from build123d import *

# Parameters (mm, degrees)
F0_W      = 63.5
F0_H      = 64
F1_DEPTH  = 2.5
F3_DEPTH  = 12
F5_DEPTH  = 10
F6_R      = 2.2
F7_R      = 2
F8_R      = 1.95
F9_DEPTH  = 1.5
F10_R     = 1.49999
F11_R     = 1.95
F12_DEPTH = 1.5
F13_R     = 1.49999


# Not quite as in the source:
# - a fillet or chamfer is up to 0.001 mm smaller than in the source, because OpenCascade refuses the exact size


with BuildPart() as f1:
    # F0 (on Top) → F1 (new body)
    with BuildSketch(Plane.XY):
        Rectangle(F0_W, F0_H)
    extrude(amount=F1_DEPTH)

    # F2 (on face) → F3 (join)
    with BuildSketch(Plane.XY.offset(2.5)):
        Polygon((-25.75, 32), (-31.75, 32), (-31.75, -32), (31.75, -32), (31.75, 32), (25.75, 32), (25.75, -26), (-25.75, -26), align=None)
    extrude(amount=F3_DEPTH)

    # F4 (on face) → F5 (join)
    with BuildSketch(Plane.XY.offset(14.5)):
        Polygon((-28.9, 32), (-31.75, 32), (-31.75, -32), (31.75, -32), (31.75, 32), (28.9, 32), (28.9, -29.15), (-28.9, -29.15), align=None)
    extrude(amount=F5_DEPTH)

    # F6
    f6_edges = [f1.edges().sort_by_distance(p)[0] for p in [
        (-28.9, -29.15, 19.5),
        (28.9, -29.15, 19.5),
    ]]
    fillet(f6_edges, radius=F6_R)

    # F7
    f7_edges = [f1.edges().sort_by_distance(p)[0] for p in [
        (-31.75, 0, 24.5),
        (0, -32, 24.5),
        (31.75, 0, 24.5),
    ]]
    fillet(f7_edges, radius=F7_R)

    # F8 (on face) → F9 (join)
    with BuildSketch(Plane.YZ.offset(-28.9)):
        with Locations((0, 19.5)):
            Circle(F8_R)
    extrude(amount=F9_DEPTH)

    # F10 (radius 1.5 in the source; OpenCascade refuses exactly that, so slightly less here)
    f10_edges = [f1.edges().sort_by_distance(p)[0] for p in [
        (-27.4, -1.95, 19.5),
    ]]
    fillet(f10_edges, radius=F10_R)

    # F11 (on face) → F12 (join)
    with BuildSketch(Plane(origin=(28.9, 0, 0), x_dir=(0, -1, 0), z_dir=(-1, 0, 0))):
        with Locations((0, 19.5)):
            Circle(F11_R)
    extrude(amount=F12_DEPTH)

    # F13 (radius 1.5 in the source; OpenCascade refuses exactly that, so slightly less here)
    f13_edges = [f1.edges().sort_by_distance(p)[0] for p in [
        (27.4, 1.95, 19.5),
    ]]
    fillet(f13_edges, radius=F13_R)


solid = f1.part
Work out the finished part from the listing and answer in its coordinate system (mm). A direction names the side the tool comes from. Coordinates: 2 decimals unless noted, no trailing zeros. Write each loop counter-clockwise with the first axis right and the second up, starting at its lowest first coordinate (ties: lowest second). Pieces come first, ordered by that corner, then holes. Notation, with made-up numbers: M 27.25,41.25 L 37.25,41.25 A14 cw 37.25,48.25 Z; hole C -28,2.5 d8. An arc over 180 degrees is marked long. Use one line per item in the form item = value. Start each with the question number.
1. The part is cut by section B-B (z = 12.5). Give the vertices of the cut face in (x, y).
2. The part is cut by section C-C (y = -9). Give the vertices of the cut face in (x, z), plus the area to 3 significant figures.
3. Straight lines are drawn through the part: probe 1 along X at (y, z) = (25, 17.75); probe 2 along X at (y, z) = (2.5, 4); probe 3 along Y at (x, z) = (-2.5, 14.25). For each, find the intervals that lie inside material, in ascending order. Write a range as from..to.
4. A tool of negligible diameter and unlimited length cuts with its end or side. For faces 1 (the face through (31.75, 0, 11)), 2 (the face through (0, 3, 2.5)), 3 (the face through (-28.24, -28.52, 19.57)), from which of +Z, -Z, +X, -X, +Y, -Y can it reach the whole face along a straight path? Write none if from no direction.
5. Each of these flat-tipped pins is pushed along its axis until it touches: P1, Ø12, axis at x = 15, z = 4, coming from the +Y side; P2, Ø6, axis at x = 4.5, z = 10, coming from the +Y side; P3, Ø10, axis at x = 19.5, y = -0.5, coming from the +Z side; P4, Ø3, axis at x = -9, z = 20, coming from the +Y side. Where does it stop, or does it pass through?
6. The part is cut by section A-A (x = 22). Give the vertices of the cut face in (y, z).
Evaluation:
q1.outline = M -31.75,-32 L 31.75,-32 L 31.75,32 L 25.75,32 L 25.75,-26 L -25.75,-26 L -25.75,32 L -31.75,32 Z
q2.outline = M -31.75,0 L 31.75,0 L 31.75,22.5 A2 ccw 29.75,24.5 L 28.9,24.5 L 28.9,14.5 L 25.75,14.5 L 25.75,2.5 L -25.75,2.5 L -25.75,14.5 L -28.9,14.5 L -28.9,24.5 L -29.75,24.5 A2 ccw -31.75,22.5 Z
q2.area = 358 mm^2
q3.probe_1 = -31.75..-28.9, 28.9..31.75
q3.probe_2 = -31.75..-25.75, 25.75..31.75
q3.probe_3 = -32..-26
q4.face_1 = +Z, -Z, +X, +Y, -Y
q4.face_2 = +Z, +Y
q4.face_3 = +Z
q5.P1 = 32
q5.P2 = -26
q5.P3 = 2.5
q5.P4 = -29.15
q6.outline = M -32,0 L 32,0 L 32,2.5 L -26,2.5 L -26,14.5 L -29.15,14.5 L -29.15,24.5 L -30,24.5 A2 ccw -32,22.5 Z
